Could you check a few things on this model? Use its own coordinates, in mm. A direction names the side the tool comes from. Give positions to 0.01 mm unless a question says otherwise; leave off trailing zeros. Order: outer loops, then holes, each group sorted by start corner. A loop starts at its lowest first (then second) coordinate and runs counter-clockwise, first axis right, second up. Notation, with made-up numbers: (1.25, 63) - (46.25, 63) arc R19 ccw to (46.25, 74) - close; hole circle Ø1 at (51.25, 22). An arc over 180 degrees is marked (long way). One line per question, with ' | ' between items. Start each with the question number.
1. Imagine slicing it at A-A (x = 0). Please give me the cut outline in (y, z), and give its area (3 significant figures).
2. Which directions (+Z, -Z, +X, -X, +Y, -Y) give clear straight access to the entire face, cutting with the end or side of a thin tool? Please do faces 1 (the cylindrical face through (-1.73, -7.81, 31.14)), 2 (the cylindrical face through (0.596, -2.685, -1.789)), 3 (the cylindrical face through (-7.678, 2.418, 0.989)), 4 (the cylindrical face through (6.78, -0.07, 63.81)), 5 (the cylindrical face through (4.08, 0.04, 63.81)).
3. I need wall thicknesses on probe 1 along X at (y, z) = (0, 3.95); probe 2 along Z at (x, y) = (4, 2.25); probe 3 along Z at (x, y) = (-2, -4). Which ranges of each line are inside material? Lowest first, please. Write a range as from..to.
4. If we mould it in two halves opening along Y, with no side actions, what happens to faces 6 (the cylindrical face through (4.2, 0, 2.7)), 7 (the cylindrical face through (2.86, -0.9, -0.52)), 8 (the flat face through (0, 0, -11.8))? For each: released by +Y, released by -Y, zero draft, split by the parting line, or undercut.
5. Imagine slicing it at B-B (z = 36). Please give me the cut outline in (x, y).
6. For P1, Ø1, axis at x = 5.5, z = 40.5, coming from the -Y side (3 decimals); P2, Ø2, axis at x = -6.5, y = -5, coming from the -Z side; P3, Ø5, axis at x = 1, z = 3, coming from the -Y side; P4, Ø1.6, axis at x = -0.5, z = -9, coming from the +Y side, each with a flat end and sliding along its axis, tell me the tip position at first contact or that it passes through.
```python
from build123d import *
from build123d.topology import SkipClean

# Parameters (mm, degrees)
SKETCH_1_R             = 8
EXTRUDE_1_DEPTH        = 61.1
EXTRUDE_2_DEPTH        = 11.8
SKETCH_3_R             = 3
EXTRUDE_3_DEPTH        = 1
SKETCH_4_R             = 2.75
EXTRUDE_4_DEPTH        = 1.6
EXTRUDE_5_DEPTH        = 0.05
EXTRUDE_5_DEPTH_BACK   = 2
SKETCH_5_R             = 8.05
HOLE_WIZARD_M2_1_D     = 1.6
HOLE_WIZARD_M2_1_DEPTH = 5.2
HOLE_WIZARD_M2_1_TIP   = 0.480688495
CHAMFER_1_SIZE         = 0.25
SKETCH1_R              = 1.5
EXTRUDE1_DEPTH         = 1.4
EXTRUDE2_DEPTH         = 5.5


with BuildPart() as part:
    # 草图1 → 拉伸1 (new body)
    with BuildSketch(Plane.XY):
        Circle(SKETCH_1_R)
    extrude(amount=EXTRUDE_1_DEPTH)

    # 草图2 → 拉伸2 (add)
    with BuildSketch(Plane(origin=(0, 0, 0), x_dir=(-1, 0, 0), z_dir=(0, 0, -1))):
        with BuildLine():
            Line((-0.748331477, 1.3), (0.748331477, 1.3))
            ThreePointArc((0.748331477, 1.3), (0, -1.5), (-0.748331477, 1.3))
        make_face()
    extrude(amount=EXTRUDE_2_DEPTH)

    # 草图3 → 拉伸3 (add)
    with BuildSketch(Plane(origin=(0, 0, 0), x_dir=(-1, 0, 0), z_dir=(0, 0, -1))):
        with Locations(Location((0, 0, 0), (0, 0, 180))):
            Circle(SKETCH_3_R)
    extrude(amount=EXTRUDE_3_DEPTH)

    # 草图4 → 拉伸4 (add)
    with BuildSketch(Plane(origin=(0, 0, -1), x_dir=(-1, 0, 0), z_dir=(0, 0, -1))):
        Circle(SKETCH_4_R)
    extrude(amount=EXTRUDE_4_DEPTH)

    # 草图5 → 拉伸5 (add, two sides: drawn at the far end of the back side and taken through both)
    with BuildSketch(Plane(origin=(0, 0, 0), x_dir=(-1, 0, 0), z_dir=(0, 0, -1)).offset(-EXTRUDE_5_DEPTH_BACK)):
        Circle(SKETCH_5_R)
    extrude(amount=EXTRUDE_5_DEPTH + EXTRUDE_5_DEPTH_BACK)

    # M2 螺纹孔1
    with Locations(Plane(origin=(5, 0, -0.05), x_dir=(-1, 0, 0), z_dir=(0, 0, -1))):
        with Locations((0, 0), (10, 0)):
            Hole(HOLE_WIZARD_M2_1_D / 2, depth=HOLE_WIZARD_M2_1_DEPTH)
            with Locations((0, 0, -(HOLE_WIZARD_M2_1_DEPTH + HOLE_WIZARD_M2_1_TIP / 2))):  # 118° drill point
                Cone(0, HOLE_WIZARD_M2_1_D / 2, HOLE_WIZARD_M2_1_TIP, mode=Mode.SUBTRACT)

    # 倒角1
    chamfer_1_edges = [part.edges().sort_by_distance(p)[0] for p in [
        (-5.8, 0, -0.05),
        (4.2, 0, -0.05),
    ]]
    chamfer(chamfer_1_edges, length=CHAMFER_1_SIZE)

    # Sketch1 → Extrude1 (add)
    with SkipClean():  # the faces are left unmerged after this step: merging them gives an invalid solid
        with BuildSketch(Plane(origin=(0, 0, -2.6), x_dir=(-1, 0, 0), z_dir=(0, 0, -1))):
            with Locations(Location((0, 0, 0), (0, 0, 119.926434867))):
                Circle(SKETCH1_R)
        extrude(amount=EXTRUDE1_DEPTH)

    # Sketch2 → Extrude2 (add)
    with SkipClean():  # the faces are left unmerged after this step: merging them gives an invalid solid
        with BuildSketch(Plane.XY.offset(61.1)):
            with BuildLine():
                ThreePointArc((4.793495579, -4.793495579), (6.779026459, 0), (4.793495579, 4.793495579))
                ThreePointArc((4.793495579, 4.793495579), (2.88430727, 4.793495579), (2.88430727, 2.88430727))
                ThreePointArc((2.88430727, 2.88430727), (4.079026459, 0), (2.88430727, -2.88430727))
                ThreePointArc((2.88430727, -2.88430727), (2.88430727, -4.793495579), (4.793495579, -4.793495579))
            make_face()
        extrude(amount=EXTRUDE2_DEPTH)


solid = part.part
```
Results found:
1) outline: (-8.05, -0.05) - (-3, -0.05) - (-3, -1) - (-2.75, -1) - (-2.75, -2.6) - (-1.5, -2.6) - (-1.5, -11.8) - (1.3, -11.8) - (1.3, -4) - (1.5, -4) - (1.5, -2.6) - (2.75, -2.6) - (2.75, -1) - (3, -1) - (3, -0.05) - (8.05, -0.05) - (8.05, 2) - (8, 2) - (8, 61.1) - (-8, 61.1) - (-8, 2) - (-8.05, 2) - close | area: 1,020 mm2
2) face 1: +Z | face 2: -Z | face 3: +Z, -Z | face 4: +Z, +X | face 5: +Z, -X
3) probe 1: x = -8..-5.8, -4.2..4.2, 5.8..8 | probe 2: z = -0.05..66.6 | probe 3: z = -0.05..61.1
4) face 6: undercut | face 7: split by the parting line | face 8: zero draft
5) outline: circle Ø16 at (0, 0)
6) P1: stops at y = -6.245 | P2: stops at z = -0.05 | P3: stops at y = -8.05 | P4: stops at y = 1.3
